Input: part model. Units: mm. Frame: model coordinates. Give positions to 0.01 mm unless a question says otherwise; leave off trailing zeros. Loops run counter-clockwise (first coordinate to the right, second up) from the corner with the lowest first, then second, coordinate; pieces in that order, holes last. Notation, with made-up numbers: M 59,66 L 77,66 A13 ccw 77,90 Z; hole C 44,51.25 d1. An arc over 180 degrees is marked long. One line per item, written item: value. Start each with the question number.
(1) Section A-A on x = 10. Output: boundary loops of the cut face in (y, z), plus the area to 3 significant figures.
(2) Section B-B on x = -70. Output: boundary loops of the cut face in (y, z), plus the area to 3 significant figures.
(3) Section C-C on y = 6.25. State how many separate pieces and enclosed holes the cut face has, plus the area to 3 significant figures.
(4) Ray query, line 1 along Y through (x, z) = (-20, -3.5) (3 decimals); line 2 along Y through (x, z) = (-31, -5.25). Return the intervals inside material, ascending. Write a range as from..to.
```python
from build123d import *

# Parameters (mm, degrees)
SKETCH1_W           = 200
SKETCH1_H           = 25
SKETCH1_R           = 3.98
SKETCH1_R_2         = 3.985
SKETCH1_R_3         = 3.99
SKETCH1_R_4         = 3.995
SKETCH1_R_5         = 4
SKETCH1_R_6         = 4.005
SKETCH1_R_7         = 4.01
SKETCH1_R_8         = 4.015
SKETCH1_R_9         = 4.02
SKETCH1_R_10        = 4.025
SKETCH1_R_11        = 4.03
SKETCH1_R_12        = 4.035
SKETCH1_R_13        = 4.04
SKETCH1_R_14        = 4.045
SKETCH1_R_15        = 4.05
SKETCH1_R_16        = 4.055
SKETCH1_R_17        = 4.06
SKETCH1_R_18        = 4.065
SKETCH1_R_19        = 4.07
BOSS_EXTRUDE1_DEPTH = 30


with BuildPart() as part:
    # Sketch1 → Boss-Extrude1 (new body)
    with BuildSketch(Plane.XY):
        Rectangle(SKETCH1_W, SKETCH1_H)
        with Locations((-90, 6.25)):
            Circle(SKETCH1_R, mode=Mode.SUBTRACT)
        with Locations((-80, 6.25)):
            Circle(SKETCH1_R_2, mode=Mode.SUBTRACT)
        with Locations((-70, 6.25)):
            Circle(SKETCH1_R_3, mode=Mode.SUBTRACT)
        with Locations((-60, 6.25)):
            Circle(SKETCH1_R_4, mode=Mode.SUBTRACT)
        with Locations((-50, 6.25)):
            Circle(SKETCH1_R_5, mode=Mode.SUBTRACT)
        with Locations((-40, 6.25)):
            Circle(SKETCH1_R_6, mode=Mode.SUBTRACT)
        with Locations((-30, 6.25)):
            Circle(SKETCH1_R_7, mode=Mode.SUBTRACT)
        with Locations((-20, 6.25)):
            Circle(SKETCH1_R_8, mode=Mode.SUBTRACT)
        with Locations((-10, 6.25)):
            Circle(SKETCH1_R_9, mode=Mode.SUBTRACT)
        with Locations((0, 6.25)):
            Circle(SKETCH1_R_10, mode=Mode.SUBTRACT)
        with Locations((10, 6.25)):
            Circle(SKETCH1_R_11, mode=Mode.SUBTRACT)
        with Locations((20, 6.25)):
            Circle(SKETCH1_R_12, mode=Mode.SUBTRACT)
        with Locations((30, 6.25)):
            Circle(SKETCH1_R_13, mode=Mode.SUBTRACT)
        with Locations((40, 6.25)):
            Circle(SKETCH1_R_14, mode=Mode.SUBTRACT)
        with Locations((50, 6.25)):
            Circle(SKETCH1_R_15, mode=Mode.SUBTRACT)
        with Locations((60, 6.25)):
            Circle(SKETCH1_R_16, mode=Mode.SUBTRACT)
        with Locations((70, 6.25)):
            Circle(SKETCH1_R_17, mode=Mode.SUBTRACT)
        with Locations((80, 6.25)):
            Circle(SKETCH1_R_18, mode=Mode.SUBTRACT)
        with Locations((90, 6.25)):
            Circle(SKETCH1_R_19, mode=Mode.SUBTRACT)
        Polygon((-91.981236116, -2.818398385), (-88.018763884, -2.818398385), (-86.037527767, -6.25), (-88.018763884, -9.681601615), (-91.981236116, -9.681601615), (-93.962472233, -6.25), align=None, mode=Mode.SUBTRACT)
        Polygon((-81.984122868, -2.813398385), (-78.015877132, -2.813398385), (-76.031754265, -6.25), (-78.015877132, -9.686601615), (-81.984122868, -9.686601615), (-83.968245735, -6.25), align=None, mode=Mode.SUBTRACT)
        Polygon((-71.987009619, -2.808398385), (-68.012990381, -2.808398385), (-66.025980762, -6.25), (-68.012990381, -9.691601615), (-71.987009619, -9.691601615), (-73.974019238, -6.25), align=None, mode=Mode.SUBTRACT)
        Polygon((-61.98989637, -2.803398385), (-58.01010363, -2.803398385), (-56.020207259, -6.25), (-58.01010363, -9.696601615), (-61.98989637, -9.696601615), (-63.979792741, -6.25), align=None, mode=Mode.SUBTRACT)
        Polygon((-51.992783122, -2.798398385), (-48.007216878, -2.798398385), (-46.014433757, -6.25), (-48.007216878, -9.701601615), (-51.992783122, -9.701601615), (-53.985566243, -6.25), align=None, mode=Mode.SUBTRACT)
        Polygon((-41.995669873, -2.793398385), (-38.004330127, -2.793398385), (-36.008660254, -6.25), (-38.004330127, -9.706601615), (-41.995669873, -9.706601615), (-43.991339746, -6.25), align=None, mode=Mode.SUBTRACT)
        Polygon((-31.998556624, -2.788398385), (-28.001443376, -2.788398385), (-26.002886751, -6.25), (-28.001443376, -9.711601615), (-31.998556624, -9.711601615), (-33.997113249, -6.25), align=None, mode=Mode.SUBTRACT)
        Polygon((-22.001443376, -2.783398385), (-17.998556624, -2.783398385), (-15.997113249, -6.25), (-17.998556624, -9.716601615), (-22.001443376, -9.716601615), (-24.002886751, -6.25), align=None, mode=Mode.SUBTRACT)
        Polygon((-12.004330127, -2.778398385), (-7.995669873, -2.778398385), (-5.991339746, -6.25), (-7.995669873, -9.721601615), (-12.004330127, -9.721601615), (-14.008660254, -6.25), align=None, mode=Mode.SUBTRACT)
        Polygon((-2.007216878, -2.773398385), (2.007216878, -2.773398385), (4.014433757, -6.25), (2.007216878, -9.726601615), (-2.007216878, -9.726601615), (-4.014433757, -6.25), align=None, mode=Mode.SUBTRACT)
        Polygon((7.98989637, -2.768398385), (12.01010363, -2.768398385), (14.020207259, -6.25), (12.01010363, -9.731601615), (7.98989637, -9.731601615), (5.979792741, -6.25), align=None, mode=Mode.SUBTRACT)
        Polygon((17.987009619, -2.763398385), (22.012990381, -2.763398385), (24.025980762, -6.25), (22.012990381, -9.736601615), (17.987009619, -9.736601615), (15.974019238, -6.25), align=None, mode=Mode.SUBTRACT)
        Polygon((27.984122868, -2.758398385), (32.015877132, -2.758398385), (34.031754265, -6.25), (32.015877132, -9.741601615), (27.984122868, -9.741601615), (25.968245735, -6.25), align=None, mode=Mode.SUBTRACT)
        Polygon((37.981236116, -2.753398385), (42.018763884, -2.753398385), (44.037527767, -6.25), (42.018763884, -9.746601615), (37.981236116, -9.746601615), (35.962472233, -6.25), align=None, mode=Mode.SUBTRACT)
        Polygon((47.978349365, -2.748398385), (52.021650635, -2.748398385), (54.04330127, -6.25), (52.021650635, -9.751601615), (47.978349365, -9.751601615), (45.95669873, -6.25), align=None, mode=Mode.SUBTRACT)
        Polygon((57.975462614, -2.743398385), (62.024537386, -2.743398385), (64.049074773, -6.25), (62.024537386, -9.756601615), (57.975462614, -9.756601615), (55.950925227, -6.25), align=None, mode=Mode.SUBTRACT)
        Polygon((67.972575862, -2.738398385), (72.027424138, -2.738398385), (74.054848276, -6.25), (72.027424138, -9.761601615), (67.972575862, -9.761601615), (65.945151724, -6.25), align=None, mode=Mode.SUBTRACT)
        Polygon((77.969689111, -2.733398385), (82.030310889, -2.733398385), (84.060621778, -6.25), (82.030310889, -9.766601615), (77.969689111, -9.766601615), (75.939378222, -6.25), align=None, mode=Mode.SUBTRACT)
        Polygon((87.96680236, -2.728398385), (92.03319764, -2.728398385), (94.066395281, -6.25), (92.03319764, -9.771601615), (87.96680236, -9.771601615), (85.933604719, -6.25), align=None, mode=Mode.SUBTRACT)
    extrude(amount=-BOSS_EXTRUDE1_DEPTH)


solid = part.part
```
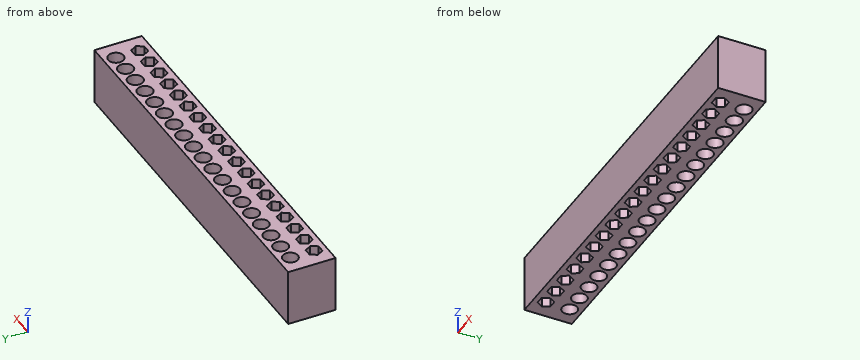
Output values:
1. outline: M -12.5,-30 L -9.73,-30 L -9.73,0 L -12.5,0 Z; M -2.77,-30 L 2.22,-30 L 2.22,0 L -2.77,0 Z; M 10.28,-30 L 12.5,-30 L 12.5,0 L 10.28,0 Z
1. area: 299 mm²
2. outline: M -12.5,-30 L -9.69,-30 L -9.69,0 L -12.5,0 Z; M -2.81,-30 L 2.26,-30 L 2.26,0 L -2.81,0 Z; M 10.24,-30 L 12.5,-30 L 12.5,0 L 10.24,0 Z
2. area: 304 mm²
3. separate pieces: 20
3. enclosed holes: 0
3. area: 1,410 mm²
4. line 1: y = -12.5..-9.717, -2.783..2.235, 10.265..12.5
4. line 2: y = -12.5..-9.71, -2.79..2.37, 10.13..12.5
